Autodesk Inventor part; units mm, degrees
ref_plane "YZ Plane" through (0, 0, 0) normal (1, 0, 0) x (0, 1, 0)
ref_plane "XZ Plane" through (0, 0, 0) normal (0, 1, 0) x (-1, 0, 0)
ref_plane "XY Plane" through (0, 0, 0) normal (0, 0, 1) x (1, 0, 0)
sketch "Skizze1" plane through (0, 0, 0) normal (0, 0, 1) x (1, 0, 0)
  line L0 (-52.5, 52.5) -> (52.5, 52.5)
  line L1 (52.5, 52.5) -> (52.5, -52.5)
  line L2 (52.5, -52.5) -> (-52.5, -52.5)
  line L3 (-52.5, -52.5) -> (-52.5, 52.5)
  line L4 (-52.5, 52.5) -> (52.5, -52.5) construction
  line L5 (52.5, 52.5) -> (-52.5, -52.5) construction
  point P0 (0, 0)
  dimension "d0" = 105
  dimension "d1" = 105
extrude "Extrusion1" add sketch "Skizze1" along normal blind 505
sketch "Skizze2" plane through (0, 0, 505) normal (0, 0, 1) x (1, 0, 0)
  spline S0 degree 3 poles (30.8941, -22.3608) (33.2455, -20.1357) (33.4278, -16.4642) (34.1009, -12.3897) (34.4408, -6.5615) (32.3239, 0.3889) (27.6464, 2.563) (18.7777, 8.3579) (6.0522, 19.3643) (-10.5838, 24.0919) (-22.9306, 22.7109) (-28.1368, 17.5955) (-28.9312, 16.6042) knots 0 0 0 0 0.05535 0.076528 0.211782 0.295547 0.382964 0.432922 0.754884 0.81234 0.967238 1 1 1 1
  spline S1 degree 3 poles (-28.9312, 16.6042) (-32.363, 12.3217) (-33.922, 4.96) (-34.2212, -5.2183) (-33.7128, -11.7973) (-30.1787, -16.4552) (-26.4199, -18.3019) (-21.7499, -13.8164) (-22.8916, -9.4321) (-23.5075, -1.7153) (-24.1566, 7.4044) (-16.6489, 14.0721) (-3.6681, 12.4997) (3.1986, 4.5284) (3.2907, 1.6248) (4.5253, 0.0908) (6.4773, -0.7371) (8.3789, 1.0013) (13.1845, -1.004) (13.6371, -9.218) (17.043, -16.25) (23.1831, -17.8066) (25.3482, -18.6226) (26.133, -19.8789) (26.5745, -22.0211) (27.7048, -23.641) (30.0236, -23.1574) (30.8172, -22.4336) (30.8941, -22.3608) knots 0 0 0 0 0.14153 0.17035 0.245987 0.25892 0.290227 0.326265 0.372233 0.38898 0.482096 0.508256 0.624416 0.647418 0.715274 0.72607 0.746892 0.801722 0.811885 0.848514 0.916356 0.943374 0.948219 0.962959 0.96651 0.98188 0.998188 1 1 1 1
  arc A0 (27.4787, -6.7498) -> (23.9934, -5.2356) centre (25, -7.687) ccw
  line L0 (27.4787, -6.7498) -> (26.0066, -10.1384)
  arc A1 (22.5213, -8.6242) -> (26.0066, -10.1384) centre (25, -7.687) ccw
  line L1 (22.5213, -8.6242) -> (23.9934, -5.2356)
  line L2 (22.5213, -8.6242) -> (23.9934, -5.2356)
  arc A2 (22.5213, -8.6242) -> (26.0066, -10.1384) centre (25, -7.687) ccw
  line L3 (27.4787, -6.7498) -> (26.0066, -10.1384)
  arc A3 (27.4787, -6.7498) -> (23.9934, -5.2356) centre (25, -7.687) ccw
  line L4 (-52.5, 52.5) -> (-52.5, -52.5) construction
  line L5 (-52.5, 0) -> (52.5, 0) construction
  line L6 (52.5, -52.5) -> (52.5, 52.5) construction
  line L7 (-34.1215, 23.4036) -> (-34.1215, -17.2518) construction
  line L8 (34.1216, 27.1841) -> (34.1216, -29.8621) construction
  line L9 (-36.6715, 23.259) -> (37.4151, 23.259) construction
  line L10 (-34.1215, -23.2592) -> (37.4151, -23.2592) construction
  point P0 (0, 0)
  point P1 (0, 0)
  dimension "d4" = 34.1215
  dimension "d6" = 34.1216
  dimension "d10" = 23.259
  dimension "d11" = 23.2592
extrude "Extrusion2" cut sketch "Skizze2" against normal blind 505 contours S1 S0 | L0 A1 L1 A0
sketch "Skizze5" plane through (0, 0, 505) normal (0, 0, 1) x (1, 0, 0)
  line L0 (-37.5, 37.5) -> (37.5, 37.5)
  line L1 (37.5, 37.5) -> (37.5, -37.5)
  line L2 (37.5, -37.5) -> (-37.5, -37.5)
  line L3 (-37.5, -37.5) -> (-37.5, 37.5)
  line L4 (-37.5, 37.5) -> (37.5, -37.5) construction
  line L5 (37.5, 37.5) -> (-37.5, -37.5) construction
  spline S0 degree 3 poles (-28.9312, 16.6042) (-28.1368, 17.5955) (-22.9306, 22.7109) (-10.5838, 24.0919) (6.0522, 19.3643) (18.7777, 8.3579) (27.6464, 2.563) (32.3239, 0.3889) (34.4408, -6.5615) (34.1009, -12.3897) (33.4278, -16.4642) (33.2455, -20.1357) (30.8941, -22.3608) knots 0 0 0 0 0.032762 0.18766 0.245116 0.567078 0.617036 0.704453 0.788218 0.923472 0.94465 1 1 1 1
  spline S1 degree 3 poles (30.8941, -22.3608) (30.8172, -22.4336) (30.0236, -23.1574) (27.7048, -23.641) (26.5745, -22.0211) (26.133, -19.8789) (25.3482, -18.6226) (23.1831, -17.8066) (17.043, -16.25) (13.6371, -9.218) (13.1845, -1.004) (8.3789, 1.0013) (6.4773, -0.7371) (4.5253, 0.0908) (3.2907, 1.6248) (3.1986, 4.5284) (-3.6681, 12.4997) (-16.6489, 14.0721) (-24.1566, 7.4044) (-23.5075, -1.7153) (-22.8916, -9.4321) (-21.7499, -13.8164) (-26.4199, -18.3019) (-30.1787, -16.4552) (-33.7128, -11.7973) (-34.2212, -5.2183) (-33.922, 4.96) (-32.363, 12.3217) (-28.9312, 16.6042) knots 0 0 0 0 0.001812 0.01812 0.03349 0.037041 0.051781 0.056626 0.083644 0.151486 0.188115 0.198278 0.253108 0.27393 0.284726 0.352582 0.375584 0.491744 0.517904 0.61102 0.627767 0.673735 0.709773 0.74108 0.754013 0.82965 0.85847 1 1 1 1
  point P0 (0, 0)
  dimension "d18" = 75
  dimension "d19" = 75
extrude "Extrusion3" cut sketch "Skizze5" against normal blind 505
sketch "Skizze8" plane through (52.5, -52.5, 0) normal (1, 0, 0) x (0, 0, -1)
  line L0 (-505, 0) -> (-505, 105)
  line L1 (0, 105) -> (-505, 105)
  line L2 (-505, 0) -> (-485, 0)
  line L3 (-485, 0) -> (-485, 105)
  line L4 (-485, 105) -> (-505, 105)
  line L5 (-505, 105) -> (-505, 0)
  point P0 (0, 52.5)
  dimension "d33" = 20
extrude "Extrusion5" cut sketch "Skizze8" against normal blind 3
mirror "Spiegeln2" about plane through (0, 0, 0) normal (1, 0, 0) of "Extrusion5"
sketch "Skizze9" plane through (49.5, -52.5, 0) normal (1, 0, 0) x (0, 0, -1)
  line L0 (-505, 0) -> (-505, 105)
  line L1 (-505, 105) -> (-485, 105)
  point P0 (0, 52.5)
  point P1 (-495, 32.5)
  point P2 (-495, 72.5)
  dimension "d36" = 10
  dimension "d37" = 40
  dimension "d38" = 32.5
hole "Bohrung2" at (49.5, -20, 495) at (49.5, 20, 495) direction (-1, 0, 0) diameter 4.917 depth 12
mirror "Spiegeln3" about plane through (0, 0, 0) normal (1, 0, 0) of "Bohrung2"
sketch "Skizze11" plane through (0, 0, 0) normal (0, 0, -1) x (-1, 0, 0)
  line L0 (52.5, 52.5) -> (52.5, -52.5)
  line L1 (52.5, -52.5) -> (-52.5, -52.5)
  point P0 (0, 0)
  point P1 (45, -45)
  dimension "d46" = 7.5
  dimension "d47" = 7.5
hole "Bohrung3" at (-45, -45, 0) direction (0, 0, 1) diameter 4.917 depth 14 tip angle 118
pattern_circular "Runde Anordnung1" count 4 over 360 about axis through (0, 0, -10) along (0, 0, 1) of "Bohrung3"
equation "\"d0\" = Magazin_Laenge"
equation "\"d1\" = Magazin_Breite"
equation "\"d2\" = Magazin_Hoehe"
equation "\"d12\" = Magazin_Hoehe"
equation "\"d18\" = Magazin_Breite - 2 * Wanddicke"
equation "\"d19\" = Magazin_Laenge - 2 * Wanddicke"
equation "\"d20\" = Magazin_Hoehe"
equation "\"d33\" = oberer_Absatz"
equation "\"Magazin_Hoehe\" = 505"
equation "\"Magazin_Laenge\" = Magazin_Breite"
equation "\"Wanddicke\" = 15"
equation "\"Bohrungsversatz_oben\" = 10"
equation "\"Bohrungsabstand_oben\" = 40"
equation "\"oberer_Absatz\" = 20"
properties part number "TS_Magazin_int"
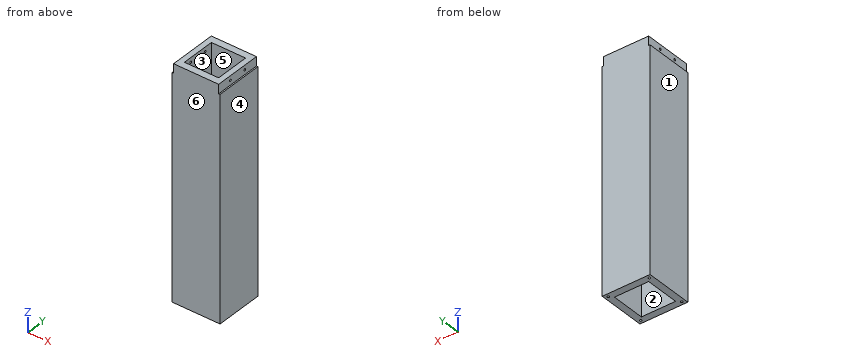
Verification items for the finished model (mm, model axes). Face numbers are marked on the shaded views. A direction names the side the tool comes from. Round coordinates to 2 decimals unless told otherwise and drop trailing zeros. Order: outer loops, then holes, each group sorted by start corner. A loop starts at its lowest first (then second) coordinate and runs counter-clockwise, first axis right, second up. Notation, with made-up numbers: (83.25, 31.25) - (106.25, 31.25) arc R28 cw to (106.25, 57.25) - close; hole circle Ø8 at (46.25, 69). An arc over 180 degrees is marked (long way). Use CSV: the item, a comma, the result in double quotes.
(1) Section check A-A on z = 334. Record the boundary of the cut face in (x, y), and give its area (3 significant figures).
Entries:
outline,"(-52.5, -52.5) - (52.5, -52.5) - (52.5, 52.5) - (-52.5, 52.5) - close; hole (-37.5, -37.5) - (37.5, -37.5) - (37.5, 37.5) - (-37.5, 37.5) - close"
area,"5,400 mm^2"
(2) Thickness scan on probe 1 along Y at (x, z) = (-46.5, 495); probe 2 along Y at (x, z) = (-45, 7.25); probe 3 along Y at (x, z) = (-22, 327). Record the ranges inside material, lowest first. Write a range as from..to.
Entries:
probe 1,"-52.5..-22.46, -17.54..17.54, 22.46..52.5"
probe 2,"-52.5..-47.46, -42.54..42.54, 47.46..52.5"
probe 3,"-52.5..-37.5, 37.5..52.5"
(3) Section check B-B on x = -14.5. Record the boundary of the cut face in (y, z), and give its area (4 significant figures).
Entries:
outline,"(-52.5, 0) - (-37.5, 0) - (-37.5, 505) - (-52.5, 505) - close; (37.5, 0) - (52.5, 0) - (52.5, 505) - (37.5, 505) - close"
area,"15,150 mm^2"
(4) Mould release check, pull along Y, two halves, no side actions. Record for the marked faces 3, 4, 5 and 6: released by +Y, released by -Y, zero draft, split by the parting line, or undercut.
Entries:
face 3,"undercut"
face 4,"zero draft"
face 5,"undercut"
face 6,"released by -Y"
(5) Access from +Z, -Z, +X, -X, +Y, -Y to the whole of each face (thin tool, end or side, straight path). Record for the marked faces 1 and 2.
Entries:
face 1,"+Z, -Z, -X, +Y, -Y"
face 2,"+Z, -Z"
(6) Gauge pin test, flat ends, axial feed: pin 1 Ø6.5 at (y, z) = (-20, 495) entering from -X; pin 2 Ø0.9 at (x, y) = (51, -15) entering from +Z; pin 3 Ø8 at (x, y) = (45, 45) entering from -Z; pin 4 Ø4 at (x, y) = (-45, -45) entering from -Z. Record the tip position at first contact, or that the pin passes through.
Entries:
pin 1,"x = -49.5"
pin 2,"z = 485"
pin 3,"z = 0"
pin 4,"z = 14.28"
